For this review, take the finished solid that the model builds, in its own axes (mm). Coordinates: 2 decimals unless noted, no trailing zeros. Loops run counter-clockwise (first coordinate to the right, second up) from the corner with the lowest first, then second, coordinate; pieces in that order, holes last. Notation, with made-up numbers: M 19.5,16.25 L 66.5,16.25 A11 ccw 66.5,23.25 Z; hole C 67,74 d5. An arc over 180 degrees is marked long. Write item = value, one per line.
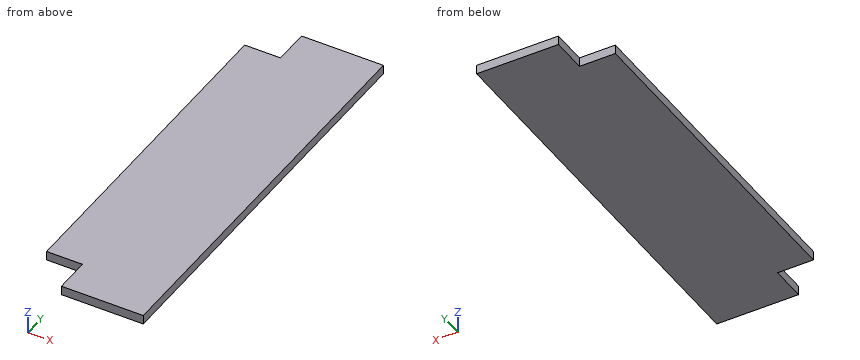
from build123d import *

# Parameters (mm, degrees)
F0_W     = 230
F0_H     = 18
F1_DEPTH = 800
F2_W     = 70
F2_H     = 70
F3_DEPTH = 18
F4_W     = 70
F4_H     = 70
F5_DEPTH = 18


with BuildPart() as f1:
    # F0 (on Front) → F1 (new body)
    with BuildSketch(Plane.XZ):
        with Locations((80.894645, 1.304673)):
            Rectangle(F0_W, F0_H)
    extrude(amount=-F1_DEPTH)

    # F2 (on face) → F3 (cut)
    with BuildSketch(Plane.XY.offset(10.304673)):
        with Locations((0.894645, 765)):
            Rectangle(F2_W, F2_H)
    extrude(amount=-F3_DEPTH, mode=Mode.SUBTRACT)

    # F4 (on face) → F5 (cut)
    with BuildSketch(Plane.XY.offset(10.304673)):
        with Locations((0.894645, 35)):
            Rectangle(F4_W, F4_H)
    extrude(amount=-F5_DEPTH, mode=Mode.SUBTRACT)


solid = f1.part
Q1. For line 1 along Y through (x, z) = (-12, -3); line 2 along X through (y, z) = (69.5, 1.5), list the stretches that pass through material, from the lowest coordinate up.
Solved:
line_1 = 70 to 730
line_2 = 35.89 to 195.89
Q2. Add section B-B (x = 13.5). Write out the cut boundary in (y, z), and give its area (3 significant figures).
Solved:
outline = M 70,-7.7 L 730,-7.7 L 730,10.3 L 70,10.3 Z
area = 11,900 mm²
Q3. For pin 1 Ø9 at (x, z) = (-7.5, 0) entering from -Y; pin 2 Ø1.5 at (x, z) = (-8.5, 5) entering from +Y; pin 3 Ø9 at (y, z) = (770.5, 3) entering from -X, all flat-tipped, find the tip position at first contact; note any pin that passes through.
Solved:
pin_1 = 70
pin_2 = 730
pin_3 = 35.89
Q4. Add section A-A (z = -3). Write out the cut boundary in (x, y), and give its area (3 significant figures).
Solved:
outline = M -34.11,70 L 35.89,70 L 35.89,0 L 195.89,0 L 195.89,800 L 35.89,800 L 35.89,730 L -34.11,730 Z
area = 174,000 mm²
